Geometry: final body of the model. Coordinates: model frame, mm. Round coordinates to 2 decimals unless told otherwise and drop trailing zeros. Loops run counter-clockwise (first coordinate to the right, second up) from the corner with the lowest first, then second, coordinate; pieces in that order, holes last. Notation, with made-up numbers: (84.5, 59.5) - (136.5, 59.5) arc R20 ccw to (136.5, 90.5) - close; hole circle Ø2 at (76.25, -9.5). An arc over 180 degrees is marked (long way). Answer in a Markdown table with one row per item. Add a question column.
Autodesk Inventor part; units mm, degrees
ref_plane "YZ Plane" through (0, 0, 0) normal (1, 0, 0) x (0, 1, 0)
ref_plane "XZ Plane" through (0, 0, 0) normal (0, 1, 0) x (-1, 0, 0)
ref_plane "XY Plane" through (0, 0, 0) normal (0, 0, 1) x (1, 0, 0)
sketch "Sketch1" plane through (0, 0, 0) normal (1, 0, 0) x (0, 1, 0)
  line L0 (12.0622, 21.4347) -> (-6.9878, 21.4347)
  line L1 (-6.9878, 21.4347) -> (-6.9878, 8.7347)
  line L2 (-6.9878, 8.7347) -> (12.0622, 8.7347)
  line L3 (12.0622, 8.7347) -> (12.0622, 21.4347)
  point P0 (0, 0)
  dimension "d0" = 12.7
  dimension "d1" = 19.05
extrude "Extrusion1" add sketch "Sketch1" along normal blind 6.858
sketch "Sketch2" plane through (6.858, 0, 0) normal (1, 0, 0) x (0, 0, -1)
  line L0 (-8.7347, -6.9878) -> (-8.7347, 12.0622)
  line L1 (-8.7347, 12.0622) -> (-21.4347, 12.0622)
  point P0 (0, 0)
  point P1 (-15.0847, 6.9822)
  point P2 (-15.0847, -1.9078)
  dimension "d4" = 6.35
  dimension "d5" = 6.35
  dimension "d6" = 13.97
  dimension "d7" = 5.08
hole "Hole1" at (6.858, 6.9822, 15.0847) at (6.858, -1.9078, 15.0847) direction (-1, 0, 0) diameter 3.175 end through all
sketch "Sketch3" plane through (6.858, 0, 0) normal (1, 0, 0) x (0, 0, -1)
  line L0 (-23.9685, 13.1299) -> (-21.0537, 13.1299)
  line L1 (-21.0537, 13.1299) -> (-21.0537, -8.0318)
  line L2 (-21.0537, -8.0318) -> (-23.9685, -8.0318)
  line L3 (-23.9685, -8.0318) -> (-23.9685, 13.1299)
  line L4 (-7.9023, 13.3864) -> (-9.1157, 13.3864)
  line L5 (-9.1157, 13.3864) -> (-9.1157, -8.3525)
  line L6 (-9.1157, -8.3525) -> (-7.9023, -8.3525)
  line L7 (-7.9023, -8.3525) -> (-7.9023, 13.3864)
  line L8 (-21.4347, 12.0622) -> (-21.4347, -6.9878)
  line L9 (-8.7347, -6.9878) -> (-8.7347, 12.0622)
  point P0 (0, 0)
  dimension "d15" = 0.381
  dimension "d16" = 0.381
extrude "Extrusion2" cut sketch "Sketch3" against normal blind 25.4
properties part number "SliderBlock"
1) Pull-direction query (Z, two-part tool) for faces 1 (the flat face through (3, 3, 21.054)), 2 (the flat face through (3, 3, 9.116)), 3 (the cylindrical face through (3.381, 7.948, 16.344)), 4 (the flat face through (0, 2, 15)); classes: pulls with the +Z half, pulls with the -Z half, needs draft (parallel to the pull), parting line crosses it, or undercut.
2) Section A-A, the plane y = -2.5. Return the cut outline in (x, z), and give its area (3 significant figures).
3) Section D-D, the plane y = 8. Return the cut outline in (x, z), and give its area (3 significant figures).
4) Section C-C, the plane x = 3.25. Return the cut outline in (y, z) (1 decimal).
5) Material intervals for line 1 along Y through (x, z) = (2.75, 16.25); line 2 along Y through (x, z) = (3, 15.5); line 3 along Z through (x, y) = (1.5, -1.25), sorted ascending. Write a range as from..to.
6) Section B-B, the plane z = 15. Return the cut outline in (x, y).
Evaluation:
| question | item | result |
|---|---|---|
| 1 | face 1 | pulls with the +Z half |
| 1 | face 2 | pulls with the -Z half |
| 1 | face 3 | undercut |
| 1 | face 4 | needs draft |
| 2 | outline | (0, 9.12) - (6.86, 9.12) - (6.86, 13.61) - (0, 13.61) - close; (0, 16.56) - (6.86, 16.56) - (6.86, 21.05) - (0, 21.05) - close |
| 2 | area | 61.7 mm² |
| 3 | outline | (0, 9.12) - (6.86, 9.12) - (6.86, 13.87) - (0, 13.87) - close; (0, 16.3) - (6.86, 16.3) - (6.86, 21.05) - (0, 21.05) - close |
| 3 | area | 65.2 mm² |
| 4 | outline | (-7, 9.1) - (12.1, 9.1) - (12.1, 21.1) - (-7, 21.1) - close; hole circle Ø3.2 at (-1.9, 15.1); hole circle Ø3.2 at (7, 15.1) |
| 5 | line 1 | y = -6.99..-2.99, -0.83..5.9, 8.06..12.06 |
| 5 | line 2 | y = -6.99..-3.44, -0.38..5.45, 8.51..12.06 |
| 5 | line 3 | z = 9.12..13.64, 16.53..21.05 |
| 6 | outline | (0, -6.99) - (6.86, -6.99) - (6.86, -3.49) - (0, -3.49) - close; (0, -0.32) - (6.86, -0.32) - (6.86, 5.4) - (0, 5.4) - close; (0, 8.57) - (6.86, 8.57) - (6.86, 12.06) - (0, 12.06) - close |
